Source: three-view drawing plus pictorial views. Frame: mm from the lowest corner of the part. Give positions to 0.01 mm unless a question says otherwise; leave off trailing zeros. Order: outer loops, then holes, each group sorted by start corner. A loop starts at its lowest first (then second) coordinate and runs counter-clockwise, first axis right, second up.
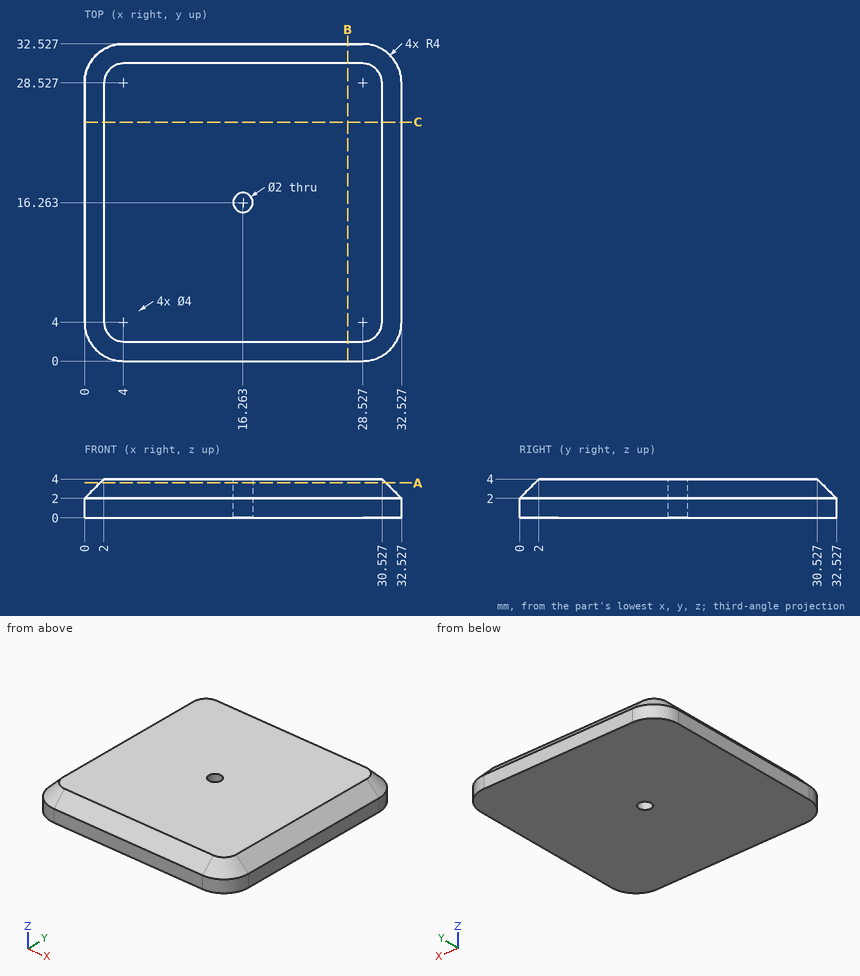
1) Section query A-A on z = 3.6. Output: boundary loops of the cut face in (x, y).
Checks:
outline: (1.6, 4) arc R2.4 ccw to (4, 1.6) - (28.53, 1.6) arc R2.4 ccw to (30.93, 4) - (30.93, 28.53) arc R2.4 ccw to (28.53, 30.93) - (4, 30.93) arc R2.4 ccw to (1.6, 28.53) - close; hole circle Ø2 at (16.26, 16.26)
2) Ray query, L1, parallel to X at y = 15.5, z = 2.7 (1 decimal); L2, parallel to X at y = 25, z = 3.2 (1 decimal); L3, parallel to X at y = 23.5, z = 3.6 (1 decimal). Return the intervals inside material, ascending.
Checks:
L1: x = 0.7 to 15.6, 16.9 to 31.8
L2: x = 1.2 to 31.3
L3: x = 1.6 to 30.9
3) Section query B-B on x = 27. Output: boundary loops of the cut face in (y, z), and give its area (3 significant figures).
Checks:
outline: (0, 0) - (32.53, 0) - (32.53, 2) - (30.53, 4) - (2, 4) - (0, 2) - close
area: 126 mm2
